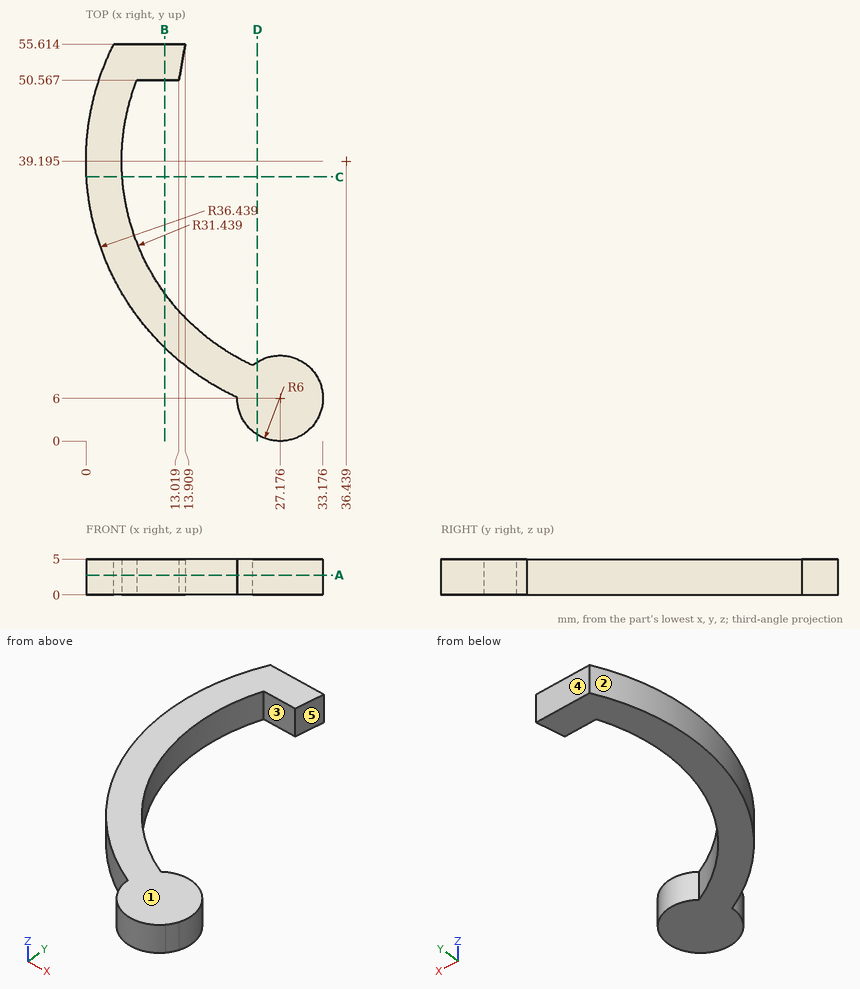
Check sheet for the drawn part. Datum: minimum x, y, z corner. Units: mm. A direction names the side the tool comes from. Give positions to 0.01 mm unless a question says otherwise; leave off trailing zeros. Loops run counter-clockwise (first coordinate to the right, second up) from the corner with the lowest first, then second, coordinate; pieces in that order, holes last. Notation, with made-up numbers: (35, 25) - (63, 25) arc R27 ccw to (63, 45) - close; hole circle Ø5 at (76, 23). An arc over 180 degrees is marked (long way). Write each question's results on one line, items separated by ' | '.
1) Material ranges on L1, parallel to X at y = 11, z = 4.45 (1 decimal); L2, parallel to X at y = 35.5, z = 1.15; L3, parallel to Y at x = 9.5, z = 0.35 (1 decimal), recorded low to high. Write a range as from..to.
Solution:
L1: 13.4..22.5, 23.9..30.5 | L2: 0.19..5.22 | L3: 14.7..23, 50.6..55.6
2) Depth check by flat-ended pin: P1, Ø1, axis at y = 44, z = 2, coming from the +X side; P2, Ø3, axis at y = 14.5, z = 2.5, coming from the -X side (1 decimal). Enter the tip coordinate at first touch or a pass-through.
Solution:
P1: x = 5.45 | P2: x = 8.3
3) Sectioned sample at B-B on x = 11. Record the boundary of the cut face in (y, z) (1 decimal).
Solution:
outline: (13.1, 0) - (20.7, 0) - (20.7, 5) - (13.1, 5) - close; (50.6, 0) - (55.6, 0) - (55.6, 5) - (50.6, 5) - close
4) Mould release check, pull along Y, two halves, no side actions. Record for the marked faces 1, 2 and 3: pulls with the +Y half, pulls with the -Y half, needs draft (parallel to the pull), parting line crosses it, or undercut.
Solution:
face 1: needs draft | face 2: parting line crosses it | face 3: undercut
5) Sectioned sample at D-D on x = 24. Record the boundary of the cut face in (y, z).
Solution:
outline: (0.91, 0) - (11.09, 0) - (11.09, 5) - (0.91, 5) - close
6) Sectioned sample at A-A on z = 2.75. Record the boundary of the cut face in (x, y) (1 decimal).
Solution:
outline: (3.9, 55.6) arc R36.4 ccw to (21.2, 6.1) arc R6 ccw (long way) to (23.3, 10.6) arc R31.4 cw to (7.1, 50.6) - (13, 50.6) - (13.9, 55.6) - close
7) Tool access check on the marked faces 4 and 5. Record the directions out of +Z, -Z, +X, -X, +Y, -Y that give a thin tool (end or side, any length) a straight path to the whole face; none if there is none.
Solution:
face 4: +Z, -Z, +X, -X, +Y | face 5: +Z, -Z, +X
8) Sectioned sample at C-C on y = 37. Record the boundary of the cut face in (x, z).
Solution:
outline: (0.07, 0) - (5.08, 0) - (5.08, 5) - (0.07, 5) - close
